Here's how the part is built. I have some questions about the finished solid (model axes, mm). Coordinates: 2 decimals unless noted, no trailing zeros. Write each loop counter-clockwise with the first axis right and the second up, starting at its lowest first coordinate (ties: lowest second). Pieces come first, ordered by that corner, then holes.
Item 1: I want a section at C-C (z = 6.5). Please give me the cut outline in (x, y).
Item 2: I want a section at D-D (x = -27.5). Please give me the cut outline in (y, z).
Item 3: Please list where these lines run through material, in increasing order: line 1 (Z direction, x = 39, y = -3.75) (3 decimals); line 2 (Z direction, x = 11, y = -0.5); line 3 (Z direction, x = -38.5, y = -6.5).
Item 4: I want a section at B-B (y = -6). Please give me the cut outline in (x, z), and give its area (3 significant figures).
Item 5: If we mould it in two halves opening along Z, with no side actions, what happens to faces 1 (the face through (15.71, -4.93, -58.45)), 2 (the face through (-54.757, -4.93, 8.741)), 3 (the face through (35.295, -4.93, -10.839)), 4 (the face through (34.52, -4.93, 16.85))? For each: pulls with the +Z half, pulls with the -Z half, needs draft (parallel to the pull), parting line crosses it, or undercut.
Item 6: I'm going to push flat-ended pins straight in: P1, Ø3, axis at y = -4.5, z = -8.5, coming from the +X side; P2, Ø5, axis at y = -8, z = -26.5, coming from the -X side; P3, Ø4, axis at y = -6.5, z = -24, coming from the +X side. Where does each tip first touch, or does it pass through?
Item 7: I want a section at A-A (x = 24.5). Please give me the cut outline in (y, z).
from build123d import *

# Parameters (mm, degrees)
F1_DEPTH = 10


with BuildPart() as f1:
    # F0 (on Front) → F1 (new body)
    with BuildSketch(Plane.XZ):
        with BuildLine():
            Line((7.292911, 3.274544), (62.522121, 30.814715))
            ThreePointArc((62.522121, 30.814715), (21.327258, 63.967445), (-30.368621, 52.847356))
            ThreePointArc((-30.368621, 52.847356), (-54.817622, 8.007093), (-37.51418, -40.044896))
            ThreePointArc((-37.51418, -40.044896), (16.53236, -58.328587), (62.523633, -24.562854))
            Line((62.523633, -24.562854), (7.292911, 3.274544))
        make_face()
    extrude(amount=F1_DEPTH)


solid = f1.part
Answer:
1. outline: (-54.92, -10) - (13.76, -10) - (13.76, 0) - (-54.92, 0) - close
2. outline: (-10, -48.48) - (0, -48.48) - (0, 54.93) - (-10, 54.93) - close
3. line 1: z = -50.175 to -12.706, 19.085 to 56.725
3. line 2: z = -58.93 to 1.41, 5.12 to 65.51
3. line 3: z = -39 to 45.46
4. outline: (-37.51, -40.04) arc R61.81 ccw to (62.52, -24.56) - (7.29, 3.27) - (62.52, 30.81) arc R61.45 ccw to (-30.37, 52.85) arc R62.29 ccw to start
4. area: 10,400 mm2
5. face 1: pulls with the -Z half
5. face 2: parting line crosses it
5. face 3: undercut
5. face 4: undercut
6. P1: stops at x = 33.63
6. P2: stops at x = -48.73
6. P3: stops at x = 62.52
7. outline: (-10, -56.55) - (0, -56.55) - (0, -5.4) - (-10, -5.4) - close; (-10, 11.85) - (0, 11.85) - (0, 63.12) - (-10, 63.12) - close
